Autodesk Inventor part; units mm, degrees
ref_plane "YZ Plane" through (0, 0, 0) normal (1, 0, 0) x (0, 1, 0)
ref_plane "XZ Plane" through (0, 0, 0) normal (0, 1, 0) x (-1, 0, 0)
ref_plane "XY Plane" through (0, 0, 0) normal (0, 0, 1) x (1, 0, 0)
sketch "Sketch2" plane through (0, 0, 0) normal (0, 1, 0) x (-1, 0, 0)
  line L0 (3.175, 0) -> (1.5875, -2.7496)
  line L1 (1.5875, -2.7496) -> (-1.5875, -2.7496)
  line L2 (-1.5875, -2.7496) -> (-3.175, 0)
  line L3 (-3.175, 0) -> (-1.5875, 2.7496)
  line L4 (-1.5875, 2.7496) -> (1.5875, 2.7496)
  line L5 (1.5875, 2.7496) -> (3.175, 0)
  point P0 (0, 0)
  point P1 (0, 0)
  dimension "d0" = 6.35
  dimension "d1" = 2.7496
extrude "Extrusion1" add sketch "Sketch2" along normal blind 25.4
sketch "Sketch3" plane through (0, 25.4, 0) normal (0, 1, 0) x (1, 0, 0)
  line L0 (-1.5875, 2.7496) -> (-3.175, 0)
  line L1 (-3.175, 0) -> (-1.5875, -2.7496)
  line L2 (-1.5875, -2.7496) -> (1.5875, -2.7496)
  line L3 (1.5875, -2.7496) -> (3.175, 0)
  line L4 (3.175, 0) -> (1.5875, 2.7496)
  line L5 (1.5875, 2.7496) -> (-1.5875, 2.7496)
  point P0 (0, 0)
hole "Hole1" at (0, 25.4, 0) direction (0, -1, 0) diameter 2.4892 end through all
properties part number "000202"
The listing builds one solid part. Answer for the finished solid, in the listing's coordinates (mm). Round coordinates to 2 decimals unless told otherwise and drop trailing zeros. Order: outer loops, then holes, each group sorted by start corner. A loop starts at its lowest first (then second) coordinate and runs counter-clockwise, first axis right, second up. Notation, with made-up numbers: M -8.5,-25 L 49.5,-25 A31 cw 49.5,5 Z; hole C 68,-14 d8. An arc over 180 degrees is marked long. Answer in a Markdown table with one row per item. Add a question column.
1) The part is cut by section C-C on z = -0.35. Determine the outline of the cut face in (x, y).
2) The part is cut by section B-B on y = 12. Determine the outline of the cut face in (x, z) (1 decimal).
3) Consider line 1 along Z through (x, y) = (0, 8.25); line 2 along X through (y, z) = (9.25, -0.2); line 3 along Z through (x, y) = (0.5, 9.25). Determine where each line is inside the solid, lowest interval first. Write a range as from..to.
4) The part is cut by section D-D on z = 1.95. Determine the outline of the cut face in (x, y).
5) Determine the mould class of faces 1 (the face through (0, 13, 2.75)), 2 (the face through (-1.4, 0, 0)), 3 (the face through (2.37, 12.522, -1.394)), 4 (the face through (-0.37, 12.52, 1.19)) for opening direction Z: pulls with the +Z half, pulls with the -Z half, needs draft (parallel to the pull), parting line crosses it, or undercut.
6) The part is cut by section A-A on x = 0. Determine the outline of the cut face in (y, z).
7) A flat-ended cylindrical pin translates along its axis: pin 1 Ø2 at (x, z) = (0, 0) entering from -Y. Find the tip coordinate at first contact, or state that the pin passes through.
Findings below:
| question | item | result |
|---|---|---|
| 1 | outline | M -2.97,0 L -1.19,0 L -1.19,25.4 L -2.97,25.4 Z; M 1.19,0 L 2.97,0 L 2.97,25.4 L 1.19,25.4 Z |
| 2 | outline | M -3.2,0 L -1.6,-2.7 L 1.6,-2.7 L 3.2,0 L 1.6,2.7 L -1.6,2.7 Z; hole C 0,0 d2.5 |
| 3 | line 1 | z = -2.75..-1.24, 1.24..2.75 |
| 3 | line 2 | x = -3.06..-1.23, 1.23..3.06 |
| 3 | line 3 | z = -2.75..-1.14, 1.14..2.75 |
| 4 | outline | M -2.05,0 L 2.05,0 L 2.05,25.4 L -2.05,25.4 Z |
| 5 | face 1 | pulls with the +Z half |
| 5 | face 2 | needs draft |
| 5 | face 3 | pulls with the -Z half |
| 5 | face 4 | undercut |
| 6 | outline | M 0,-2.75 L 25.4,-2.75 L 25.4,-1.24 L 0,-1.24 Z; M 0,1.24 L 25.4,1.24 L 25.4,2.75 L 0,2.75 Z |
| 7 | pin 1 | passes through |
